Read the model definition and answer for the solid it produces. Units are mm, in the model's axes. A direction names the side the tool comes from. Round coordinates to 2 decimals unless told otherwise and drop trailing zeros. Write each loop counter-clockwise with the first axis right and the second up, starting at its lowest first coordinate (ties: lowest second). Pieces come first, ordered by that corner, then holes. Notation, with made-up numbers: (21.5, 55.25) - (64.5, 55.25) arc R18 ccw to (64.5, 87.25) - close; hole circle Ø2 at (25, 58). An arc over 180 degrees is marked (long way). Use one line per item in the form item = value. Start each with the question number.
1) The part is cut by section C-C, the plane z = 12. Give the vertices of the cut face in (x, y) (3 decimals).
2) Each of these flat-tipped pins is pushed along its axis until it touches: pin 1 (6 mm diameter, centred on x = -48.5, z = -34, fed in from -Y); pin 2 (3 mm diameter, centred on y = -4, z = 34.5, fed in from +X). Where does it stop, or does it pass through?
3) Consider line 1 along Z through (x, y) = (81, -0.25); line 2 along X through (y, z) = (-2.35, 17); line 3 along X through (y, z) = (-2.3, 1). Determine where each line is inside the solid, lowest interval first. Write a range as from..to.
4) The part is cut by section D-D, the plane z = -44.5. Give the vertices of the cut face in (x, y).
5) The part is cut by section A-A, the plane x = 11.5. Give the vertices of the cut face in (y, z).
6) The part is cut by section B-B, the plane y = -3.8. Give the vertices of the cut face in (x, z) (3 decimals).
7) For faces 1 (the face through (-99.476, -2.465, 46.167)), 2 (the face through (96.525, -2.465, -14.579)), determine the directions among +Z, -Z, +X, -X, +Y, -Y from which every point of the face is accessible in a straight line to the end or side of a thin tool.
8) For a pull along Z with two mould halves and no side action, classify faces 3 (the face through (1, -2, -36.75)), 4 (the face through (-1, -2, 36.75)), 5 (the face through (-1, -2, -51.75)), 6 (the face through (8, 0, -38)) as released by +Z, released by -Z, zero draft, split by the parting line, or undercut.
from build123d import *

# Parameters (mm, degrees)
F1_DEPTH = 5


with BuildPart() as f1:
    # F0 (on Front) → F1 (new body)
    with BuildSketch(Plane.XZ):
        with BuildLine():
            ThreePointArc((108.329796, 31.749), (99.646478, 46.114594), (83.834694, 51.75))
            Line((83.834694, 51.75), (-83.728488, 51.75))
            ThreePointArc((-83.728488, 51.75), (-99.662707, 46.013973), (-108.284997, 31.438053))
            Line((-108.284997, 31.438053), (-113.835649, 2.36316))
            Line((-113.835649, 2.36316), (-114.243014, 0.229341))
            ThreePointArc((-114.243014, 0.229341), (-114.38477, -1.321549), (-114.223364, -2.870517))
            Line((-114.223364, -2.870517), (-113.788979, -4.999))
            Line((-113.788979, -4.999), (-108.329796, -31.749))
            ThreePointArc((-108.329796, -31.749), (-99.646478, -46.114594), (-83.834694, -51.75))
            Line((-83.834694, -51.75), (83.834694, -51.75))
            ThreePointArc((83.834694, -51.75), (99.646478, -46.114594), (108.329796, -31.749))
            Line((108.329796, -31.749), (114.033828, -3.79924))
            Line((114.033828, -3.79924), (114.482718, -1.59968))
            ThreePointArc((114.482718, -1.59968), (114.644286, 0), (114.482718, 1.59968))
            Line((114.482718, 1.59968), (114.033828, 3.79924))
            Line((114.033828, 3.79924), (109.970639, 23.708868))
            Line((109.970639, 23.708868), (108.329796, 31.749))
        make_face()
        with BuildLine():
            Line((-83.728488, 36.75), (83.834694, 36.75))
            ThreePointArc((83.834694, 36.75), (90.159407, 34.495838), (93.632735, 28.7496))
            Line((93.632735, 28.7496), (99.336767, 0.79984))
            ThreePointArc((99.336767, 0.79984), (99.417551, 0), (99.336767, -0.79984))
            Line((99.336767, -0.79984), (93.632735, -28.7496))
            ThreePointArc((93.632735, -28.7496), (90.159407, -34.495838), (83.834694, -36.75))
            Line((83.834694, -36.75), (-83.834694, -36.75))
            ThreePointArc((-83.834694, -36.75), (-90.159407, -34.495838), (-93.632735, -28.7496))
            Line((-93.632735, -28.7496), (-99.091918, -1.9996))
            ThreePointArc((-99.091918, -1.9996), (-99.172622, -1.225116), (-99.101744, -0.449672))
            Line((-99.101744, -0.449672), (-93.551092, 28.625221))
            ThreePointArc((-93.551092, 28.625221), (-90.102175, 34.455589), (-83.728488, 36.75))
        make_face(mode=Mode.SUBTRACT)
    extrude(amount=F1_DEPTH)


solid = f1.part
Geometry results:
q1.outline = (-111.996, -5) - (-96.725, -5) - (-96.725, 0) - (-111.996, 0) - close; (97.051, -5) - (112.36, -5) - (112.36, 0) - (97.051, 0) - close
q2.pin_1 = -5
q2.pin_2 = 108.04
q3.line_1 = -51.75..-36.75, 36.75..51.75
q3.line_2 = -111.04..-95.77, 96.03..111.34
q3.line_3 = -114.1..-98.82, 99.3..114.58
q4.outline = (-101.44, -5) - (101.44, -5) - (101.44, 0) - (-101.44, 0) - close
q5.outline = (-5, -51.75) - (0, -51.75) - (0, -36.75) - (-5, -36.75) - close; (-5, 36.75) - (0, 36.75) - (0, 51.75) - (-5, 51.75) - close
q6.outline = (-114.243, 0.229) arc R8 ccw to (-114.223, -2.871) - (-113.789, -4.999) - (-108.33, -31.749) arc R25 ccw to (-83.835, -51.75) - (83.835, -51.75) arc R25 ccw to (108.33, -31.749) - (114.034, -3.799) - (114.483, -1.6) arc R8 ccw to (114.483, 1.6) - (114.034, 3.799) - (108.33, 31.749) arc R25 ccw to (83.835, 51.75) - (-83.728, 51.75) arc R25 ccw to (-108.285, 31.438) - (-113.836, 2.363) - close; hole (-99.102, -0.45) arc R4 ccw to (-99.092, -2) - (-93.633, -28.75) arc R10 ccw to (-83.835, -36.75) - (83.835, -36.75) arc R10 ccw to (93.633, -28.75) - (99.337, -0.8) arc R4 ccw to (99.337, 0.8) - (93.633, 28.75) arc R10 ccw to (83.835, 36.75) - (-83.728, 36.75) arc R10 ccw to (-93.551, 28.625) - close
q7.face_1 = +Z, -X, +Y, -Y
q7.face_2 = +Y, -Y
q8.face_3 = undercut
q8.face_4 = undercut
q8.face_5 = released by -Z
q8.face_6 = zero draft
